Could you check a few things on this model? Use its own coordinates, in mm. Face numbers are marked on the shaded views. A direction names the side the tool comes from. Give positions to 0.01 mm unless a question says otherwise; leave off trailing zeros. Order: outer loops, then holes, each group sorted by start corner. A loop starts at its lowest first (then second) coordinate and runs counter-clockwise, first axis right, second up. Notation, with made-up numbers: (34.25, 61.25) -> (56.25, 61.25) arc R30 cw to (56.25, 92.25) -> close; hole circle Ø11 at (-4.75, 26.25). An arc over 180 degrees is marked (long way). Answer as CSV lines item,"result". Start each with the question number.
(1) I want a section at D-D (y = 13). Please give me the cut outline in (x, z).
(2) Will these pins go through, and if not, where does the flat tip stop? pin 1 Ø5 at (x, y) = (13.5, 31.5) entering from -Z; pin 2 Ø1.1 at (x, z) = (8, 5.5) entering from +Y; pin 3 Ø2 at (x, y) = (-14, 25) entering from +Z.
(3) On a 3-axis mill with a long thin cutter (end or side, diameter ignored), from which of +Z, -Z, +X, -X, +Y, -Y can I reach the whole of each face in a straight line? I mean the marked faces 5, 6 and 7. Say none if no direction works.
(4) I need wall thicknesses on L1, parallel to X at y = 16, z = 1.75; L2, parallel to Y at x = 7, z = 2.15; L3, parallel to X at y = 23.5, z = 5.45. Which ranges of each line are inside material? Lowest first, please.
(5) We'd pull the mould along X, two halves only. Please class the marked faces 1, 2, 3 and 4: released by +X, released by -X, zero draft, split by the parting line, or undercut.
(6) I want a section at A-A (z = 1.5). Please give me the cut outline in (x, y), plus the area to 3 significant figures.
(7) I want a section at C-C (x = 5). Please give me the cut outline in (y, z).
(8) I want a section at B-B (y = 4). Please give me the cut outline in (x, z), plus the area to 3 significant figures.
```python
from build123d import *

# Parameters (mm, degrees)
SKETCH_W        = 41.5
SKETCH_H        = 36
PAD_DEPTH       = 6
POCKET_DEPTH    = 5
SKETCH002_W     = 19.5
SKETCH002_H     = 8
POCKET001_DEPTH = 6.001
POCKET002_DEPTH = 1
SKETCH005_W     = 1
SKETCH005_H     = 19
PAD001_DEPTH    = 4
FILLET_R        = 1
FILLET001_R     = 0.4


with BuildPart() as part:
    # Sketch → Pad (new body)
    with BuildSketch(Plane.XY):
        with Locations((-0.25, 18)):
            Rectangle(SKETCH_W, SKETCH_H)
    extrude(amount=PAD_DEPTH)

    # Sketch001 (on Face6 of Pad) → Pocket (cut)
    with BuildSketch(Plane.XY.offset(6)):
        Polygon((-19, 2), (18.5, 2), (18.5, 26), (-1, 26), (-1, 34), (-19, 34), align=None)
    extrude(amount=-POCKET_DEPTH, mode=Mode.SUBTRACT)

    # Sketch002 (on Face5 of Pocket) → Pocket001 (cut, through all)
    with BuildSketch(Plane.XY.offset(6)):
        with Locations((10.75, 32)):
            Rectangle(SKETCH002_W, SKETCH002_H)
    extrude(amount=-POCKET001_DEPTH, mode=Mode.SUBTRACT)

    # Sketch004 (on Face5 of Pocket001) → Pocket002 (cut)
    with BuildSketch(Plane.XY.offset(6)):
        Polygon((-20, 35), (0, 35), (0, 27), (19.5, 27), (19.5, 1), (-20, 1), align=None)
    extrude(amount=-POCKET002_DEPTH, mode=Mode.SUBTRACT)

    # Sketch005 (on Face22 of Pocket002) → Pad001 (join)
    with BuildSketch(Plane.XY.offset(1)):
        with Locations((-0.5, 16.5)):
            Rectangle(SKETCH005_W, SKETCH005_H)
    extrude(amount=PAD001_DEPTH)

    # Fillet
    fillet_edges = [part.edges().sort_by_distance(p)[0] for p in [
        (-21, 0, 3),
        (20.5, 0, 3),
        (20.5, 28, 3),
        (1, 28, 3),
        (1, 36, 3),
        (-21, 36, 3),
    ]]
    fillet(fillet_edges, radius=FILLET_R)

    # Fillet001
    fillet001_edges = [part.edges().sort_by_distance(p)[0] for p in [
        (20.5, 14, 6),
        (20.207107, 0.292893, 6),
        (-0.25, 0, 6),
        (20.207107, 27.707107, 6),
        (10.75, 28, 6),
        (1.292893, 28.292893, 6),
        (1, 32, 6),
        (0.707107, 35.707107, 6),
        (-10, 36, 6),
        (-21, 18, 6),
        (-20.707107, 0.292893, 6),
    ]]
    fillet(fillet001_edges, radius=FILLET001_R)


solid = part.part
```
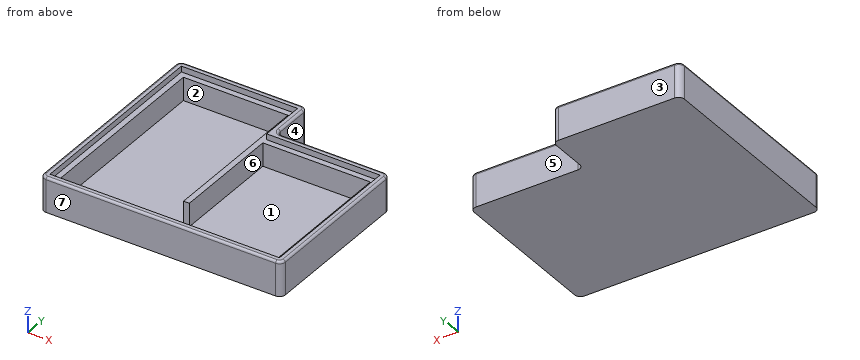
Final values:
1,outline,"(-21, 0) -> (20.5, 0) -> (20.5, 5.6) arc R0.4 ccw to (20.1, 6) -> (19.5, 6) -> (19.5, 5) -> (18.5, 5) -> (18.5, 1) -> (0, 1) -> (0, 5) -> (-1, 5) -> (-1, 1) -> (-19, 1) -> (-19, 5) -> (-20, 5) -> (-20, 6) -> (-20.6, 6) arc R0.4 ccw to (-21, 5.6) -> close"
2,pin 1,"through"
2,pin 2,"y = 28"
2,pin 3,"z = 1"
3,face 5,"+Z, -Z, +X, +Y"
3,face 6,"+Z"
3,face 7,"+Z, -Z, +X, -X, -Y"
4,L1,"-21 to -19, -1 to 0, 18.5 to 20.5"
4,L2,"0 to 2, 26 to 28"
4,L3,"-21 to -20, 19.5 to 20.5"
5,face 1,"undercut"
5,face 2,"undercut"
5,face 3,"zero draft"
5,face 4,"released by +X"
6,outline,"(-21, 1) arc R1 ccw to (-20, 0) -> (19.5, 0) arc R1 ccw to (20.5, 1) -> (20.5, 27) arc R1 ccw to (19.5, 28) -> (2, 28) arc R1 cw to (1, 29) -> (1, 35) arc R1 ccw to (0, 36) -> (-20, 36) arc R1 ccw to (-21, 35) -> close; hole (-19, 2) -> (18.5, 2) -> (18.5, 26) -> (0, 26) -> (0, 7) -> (-1, 7) -> (-1, 34) -> (-19, 34) -> close"
6,area,"312 mm²"
7,outline,"(0, 0) -> (28, 0) -> (28, 5.6) arc R0.4 ccw to (27.6, 6) -> (27, 6) -> (27, 5) -> (26, 5) -> (26, 1) -> (2, 1) -> (2, 5) -> (1, 5) -> (1, 6) -> (0.4, 6) arc R0.4 ccw to (0, 5.6) -> close"
8,outline,"(-21, 0) -> (20.5, 0) -> (20.5, 5.6) arc R0.4 ccw to (20.1, 6) -> (19.5, 6) -> (19.5, 5) -> (18.5, 5) -> (18.5, 1) -> (-19, 1) -> (-19, 5) -> (-20, 5) -> (-20, 6) -> (-20.6, 6) arc R0.4 ccw to (-21, 5.6) -> close"
8,area,"59.4 mm²"
